```python
from build123d import *

# Parameters (mm, degrees)
F1_DEPTH = 20
F2_W     = 20
F2_H     = 35
F3_DEPTH = 70
F4_W     = 30
F4_H     = 10
F5_DEPTH = 20.001


with BuildPart() as f1:
    # F0 (on Top) → F1 (new body)
    with BuildSketch(Plane.XY):
        Polygon((-47.5, -35), (47.5, -35), (47.5, -10), (7.5, -10), (7.5, 0), (7.5, 10), (47.5, 10), (47.5, 35), (-47.5, 35), align=None)
    extrude(amount=F1_DEPTH)

    # F2 (on face) → F3 (join)
    with BuildSketch(Plane.XZ.offset(35)):
        with Locations((-37.5, 37.5)):
            Rectangle(F2_W, F2_H)
    extrude(amount=-F3_DEPTH)

    # F4 (on face) → F5 (cut, through all)
    with BuildSketch(Plane.YZ.offset(-27.5)):
        with Locations((0, 50)):
            Rectangle(F4_W, F4_H)
    extrude(amount=-F5_DEPTH, mode=Mode.SUBTRACT)


solid = f1.part
```
Part model, mm, in its own coordinate system. A direction names the side the tool comes from. Give positions to 0.01 mm unless a question says otherwise; leave off trailing zeros. Order: outer loops, then holes, each group sorted by start corner. A loop starts at its lowest first (then second) coordinate and runs counter-clockwise, first axis right, second up. Notation, with made-up numbers: M -39.75,46 L 0.25,46 A26 cw 0.25,67 Z; hole C 14,16 d2. An arc over 180 degrees is marked long. Use a Markdown table: item, result. Add a question column.
(1) Saw through at D-D, the plane z = 5. Give the cut face in (x, y), and give its area (3 significant figures).
(2) Saw through at B-B, the plane z = 47.5. Give the cut face in (x, y), and give its area (3 significant figures).
(3) 3-axis set-ups, long thin cutter, end or side, ignore diameter. For faces 4 (the face through (28, -10, 10)), 5 (the face through (-27.5, 0, 37)), 6 (the face through (-37, -15, 50)), 7 (the face through (-38, -25, 55)): which of +Z, -Z, +X, -X, +Y, -Y reach the whole face in a straight line?
(4) Probe line 1 along Z through (x, y) = (35.5, -25); line 2 along Y through (x, z) = (18, 4); line 3 along X through (y, z) = (-4.5, 10). List the from-to ranges inside material, lowest first. Write a range as [from, to].
(5) Saw through at A-A, the plane x = 36. Give the cut face in (y, z).
(6) Drop flat-ended pins along their axis: P1, Ø6, axis at x = -40.5, y = 3, coming from the +Z side; P2, Ø3, axis at x = -19.5, y = 10.5, coming from the +Z side; P3, Ø3, axis at y = 8, z = 25, coming from the +X side; P4, Ø5, axis at x = -24.5, z = 40.5, coming from the -Y side. Give the stop position or say it passes through.
(7) Mould opens along Y. For faces 1 (the face through (47.5, -23, 10)), 2 (the face through (-11, 35, 16)), 3 (the face through (27, 10, 10)) say: +Y half, -Y half, draft (parallel to the pull), parting line (faces both ways), or undercut.
(8) Saw through at C-C, the plane y = 23.5. Give the cut face in (x, z), and give its area (3 significant figures).
Answer key:
| question | item | result |
|---|---|---|
| 1 | outline | M -47.5,-35 L 47.5,-35 L 47.5,-10 L 7.5,-10 L 7.5,10 L 47.5,10 L 47.5,35 L -47.5,35 Z |
| 1 | area | 5,850 mm^2 |
| 2 | outline | M -47.5,-35 L -27.5,-35 L -27.5,-15 L -47.5,-15 Z; M -47.5,15 L -27.5,15 L -27.5,35 L -47.5,35 Z |
| 2 | area | 800 mm^2 |
| 3 | face 4 | +Z, -Z, +X |
| 3 | face 5 | +Z, +X, +Y, -Y |
| 3 | face 6 | +Z, +X, -X |
| 3 | face 7 | +Z, +X, -X, +Y, -Y |
| 4 | line 1 | [0, 20] |
| 4 | line 2 | [-35, -10], [10, 35] |
| 4 | line 3 | [-47.5, 7.5] |
| 5 | outline | M -35,0 L -10,0 L -10,20 L -35,20 Z; M 10,0 L 35,0 L 35,20 L 10,20 Z |
| 6 | P1 | z = 45 |
| 6 | P2 | z = 20 |
| 6 | P3 | x = -27.5 |
| 6 | P4 | through |
| 7 | face 1 | draft |
| 7 | face 2 | +Y half |
| 7 | face 3 | undercut |
| 8 | outline | M -47.5,0 L 47.5,0 L 47.5,20 L -27.5,20 L -27.5,55 L -47.5,55 Z |
| 8 | area | 2,600 mm^2 |
